from build123d import *

# Parameters (mm, degrees)
SKETCH1_R           = 15
BOSS_EXTRUDE1_DEPTH = 503
CHAMFER1_SIZE       = 2
SKETCH2_R           = 5.177936305
CUT_EXTRUDE1_DEPTH  = 5
CHAMFER2_SIZE       = 5


with BuildPart() as part:
    # Sketch1 → Boss-Extrude1 (new body)
    with BuildSketch(Plane.XY):
        Circle(SKETCH1_R)
    extrude(amount=BOSS_EXTRUDE1_DEPTH)

    # Chamfer1
    chamfer1_edges = [part.edges().sort_by_distance(p)[0] for p in [
        (-15, 0, 503),
    ]]
    chamfer(chamfer1_edges, length=CHAMFER1_SIZE)

    # Sketch2 → Cut-Extrude1 (cut)
    with BuildSketch(Plane.XY.offset(503)):
        Circle(SKETCH2_R)
    extrude(amount=-CUT_EXTRUDE1_DEPTH, mode=Mode.SUBTRACT)

    # Chamfer2
    chamfer2_edges = [part.edges().sort_by_distance(p)[0] for p in [
        (-5.177936305, 0, 498),
    ]]
    chamfer(chamfer2_edges, length=CHAMFER2_SIZE - 0.0001)  # a hair under: the kernel refuses the full size

    # Fillet1: read off the stored shape, not the designer's step
    # Fillet1 outline → Fillet1 (revolve, cut)
    with BuildSketch(Plane.XZ):
        with BuildLine():
            ThreePointArc((14.707106781, 501.292893219), (14.923879533, 500.96846987), (15, 500.585786438))
            Line((15, 500.585786438), (15, 501.292893219))
            Line((15, 501.292893219), (14.707106781, 501.292893219))
        make_face()
        with BuildLine():
            ThreePointArc((12.585786438, 503), (12.96846987, 502.923879533), (13.292893219, 502.707106781))
            Line((13.292893219, 502.707106781), (13.292893219, 503))
            Line((13.292893219, 503), (12.585786438, 503))
        make_face()
        with BuildLine():
            ThreePointArc((4.885043086, 502.707106781), (5.209466435, 502.923879533), (5.592149867, 503))
            Line((5.592149867, 503), (4.885043086, 503))
            Line((4.885043086, 503), (4.885043086, 502.707106781))
        make_face()
    revolve(axis=Axis((0, 0, 0), (0, 0, 1)), mode=Mode.SUBTRACT)


solid = part.part
Geometry: final body of the model. Coordinates: model frame, mm. Coordinates: 2 decimals unless noted, no trailing zeros. Order: outer loops, then holes, each group sorted by start corner. A loop starts at its lowest first (then second) coordinate and runs counter-clockwise, first axis right, second up.
(1) Material intervals for probe 1 along X at (y, z) = (-2.5, 90); probe 2 along X at (y, z) = (-1.5, 289); probe 3 along Y at (x, z) = (-3, 52), sorted ascending.
(2) Section query A-A (z = 314.5). Return the cut outline in (x, y).
(3) Draft query along Y for faces 1 (the face through (3, -5, 503)), 2 (the face through (-1.155, -0.885, 499.277)), 3 (the face through (-14.985, 0.66, 246.789)). Return one class per face: pulls with the +Y half, pulls with the -Y half, needs draft (parallel to the pull), parting line crosses it, or undercut.
(4) First-contact query: pin 1 (1.5 mm diameter, centred on x = 1.5, z = 100.5, fed in from -Y); pin 2 (1.5 mm diameter, centred on x = 9.5, z = 240, fed in from +Y); pin 3 (4 mm diameter, centred on y = 9.5, z = 400.5, fed in from -X). Flat tips, straight axial feed; report the tip coordinate or a pass-through.
Solution:
1. probe 1: x = -14.79 to 14.79
1. probe 2: x = -14.92 to 14.92
1. probe 3: y = -14.7 to 14.7
2. outline: circle Ø30 at (0, 0)
3. face 1: needs draft
3. face 2: undercut
3. face 3: parting line crosses it
4. pin 1: stops at y = -14.98
4. pin 2: stops at y = 12.18
4. pin 3: stops at x = -12.99
